Model file for the job. Use its own axes, mm. Coordinates: 2 decimals unless noted, no trailing zeros. Loops run counter-clockwise (first coordinate to the right, second up) from the corner with the lowest first, then second, coordinate; pieces in that order, holes last. Notation, with made-up numbers: (-7, 11) -> (32, 11) arc R24 cw to (32, 29) -> close; hole circle Ø5 at (37.25, -3). An arc over 180 degrees is marked (long way). Use one line per item in the form item = value.
Autodesk Inventor part; units mm, degrees
ref_plane "YZ Plane" through (0, 0, 0) normal (1, 0, 0) x (0, 1, 0)
ref_plane "XZ Plane" through (0, 0, 0) normal (0, 1, 0) x (-1, 0, 0)
ref_plane "XY Plane" through (0, 0, 0) normal (0, 0, 1) x (1, 0, 0)
sketch "Sketch1" plane through (0, 0, 0) normal (0, 0, 1) x (1, 0, 0)
  line L0 (-200, 20) -> (80, 20)
  line L1 (80, 20) -> (80, -140)
  line L2 (80, -140) -> (-200, -140)
  line L3 (-200, -140) -> (-200, 20)
  point P0 (0, 0)
  dimension "d0" = 280
  dimension "d1" = 160
  dimension "d2" = 80
  dimension "d3" = 140
extrude "Extrusion1" add sketch "Sketch1" along normal blind 5
sketch "Sketch2" plane through (0, 0, 5) normal (0, 0, 1) x (1, 0, 0)
  circle A0 centre (-170, -10) radius 2.5
  point P0 (0, 0)
  point P1 (-87.5, -7.5)
  point P2 (-170, -10)
  point P3 (-170, -110)
  point P4 (-87.5, -112.5)
  point P5 (-75, -109.875)
  point P6 (-75, -94.875)
  point P7 (-75, -24.875)
  point P8 (-75, -9.875)
  point P9 (-39.999, -60)
  point P10 (30.0009, -79.878)
  point P11 (30.0009, -64.878)
  point P12 (30.0008, -54.872)
  point P13 (30.0008, -39.872)
hole "TornillosGripper" at (-87.5, -7.5, 5) at (-170, -10, 5) at (-170, -110, 5) at (-87.5, -112.5, 5) at (-75, -109.875, 5) at (-75, -94.875, 5) at (-75, -24.875, 5) at (-75, -9.875, 5) at (-39.999, -60, 5) at (30.0009, -79.878, 5) at (30.0009, -64.878, 5) at (30.0008, -54.872, 5) at (30.0008, -39.872, 5) direction (0, 0, -1) diameter 8.5 end through all
sketch "Sketch3" plane through (0, 0, 5) normal (0, 0, 1) x (1, 0, 0)
  line L0 (80, 20) -> (-200, 20)
  line L1 (-60, 20) -> (-60, -140) construction
  line L2 (-200, -140) -> (80, -140)
  line L3 (-200, 20) -> (-200, -140)
  line L4 (-200, -60) -> (80, -60) construction
  line L5 (80, -140) -> (80, 20)
  point P0 (0, 0)
  point P1 (-190, 10)
  point P2 (-190, -130)
  point P3 (70, -130)
  point P4 (70, 10)
  point P5 (50, 10)
  point P6 (50, -130)
  dimension "d13" = 10
  dimension "d14" = 10
  dimension "d22" = 20
  dimension "d23" = 10
hole "TornillosBase" at (-190, 10, 5) at (-190, -130, 5) at (70, -130, 5) at (70, 10, 5) at (50, 10, 5) at (50, -130, 5) direction (0, 0, -1) diameter 5 end through all
properties part number "BaseEnsamble" material "MDF Medium Density Fiberboard"
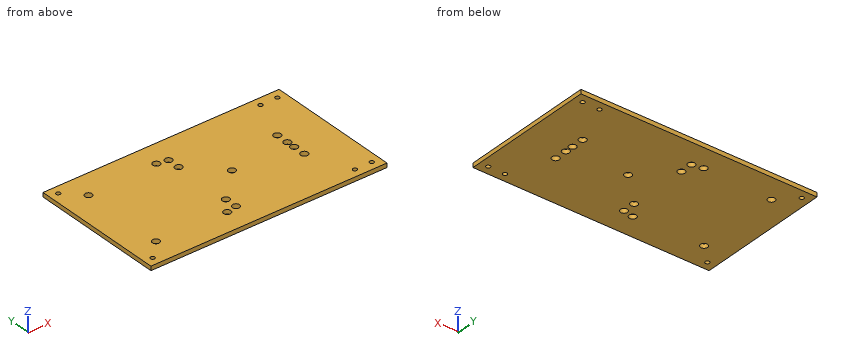
Q1. Pin check, flat tip, straight feed: pin 1 Ø3 at (x, y) = (-190, -130) entering from -Z. Stop position of the tip, or through.
Result:
pin_1 = through
Q2. Band-saw the part on A-A, the plane x = -75. Write the cut outline in (y, z) (3 decimals).
Result:
outline = (-140, 0) -> (-114.125, 0) -> (-114.125, 5) -> (-140, 5) -> close; (-105.625, 0) -> (-99.125, 0) -> (-99.125, 5) -> (-105.625, 5) -> close; (-90.625, 0) -> (-29.125, 0) -> (-29.125, 5) -> (-90.625, 5) -> close; (-20.625, 0) -> (-14.125, 0) -> (-14.125, 5) -> (-20.625, 5) -> close; (-5.625, 0) -> (20, 0) -> (20, 5) -> (-5.625, 5) -> close
Q3. Band-saw the part on B-B, the plane y = -24. Write the cut outline in (x, z).
Result:
outline = (-200, 0) -> (-79.16, 0) -> (-79.16, 5) -> (-200, 5) -> close; (-70.84, 0) -> (80, 0) -> (80, 5) -> (-70.84, 5) -> close
Q4. Wall check: line 1 along Y through (x, z) = (30.5, 4.4); line 2 along Y through (x, z) = (70, 4); line 3 along Y through (x, z) = (-170, 3.5). Give the ranges that are in metal, low to high.
Result:
line_1 = -140 to -84.1, -75.66 to -69.1, -60.66 to -59.09, -50.65 to -44.09, -35.65 to 20
line_2 = -140 to -132.5, -127.5 to 7.5, 12.5 to 20
line_3 = -140 to -114.25, -105.75 to -14.25, -5.75 to 20
Q5. Band-saw the part on C-C, the plane z = 3.35. State how many separate pieces and enclosed holes the cut face has, and give its area (3 significant figures).
Result:
separate_pieces = 1
enclosed_holes = 19
area = 43,900 mm2
